Part model, mm, in its own coordinate system. A direction names the side the tool comes from. Give positions to 0.01 mm unless a question says otherwise; leave off trailing zeros. Write each loop counter-clockwise with the first axis right and the second up, starting at its lowest first coordinate (ties: lowest second). Pieces come first, ordered by that corner, then holes.
```python
from build123d import *

# Parameters (mm, degrees)
EXTRUDE_1_DEPTH = 14
EXTRUDE_2_DEPTH = 12
SKETCH_8_W      = 500
SKETCH_8_H      = 12
EXTRUDE_5_DEPTH = 78


with BuildPart() as part:
    # 草图1 → 凸台-拉伸1 (new body)
    with BuildSketch(Plane.XY):
        Polygon((0, 0), (250, 0), (250, 50), (100, 240), (100, 340), (0, 340), (-100, 340), (-100, 240), (-250, 50), (-250, 0), align=None)
    extrude(amount=EXTRUDE_1_DEPTH)

    # 草图6 → 凸台-拉伸2 (add)
    with BuildSketch(Plane.XY.offset(14)):
        Polygon((218.421052632, 90), (-218.421052632, 90), (-250, 50), (-250, 0), (250, 0), (250, 50), align=None)
    extrude(amount=EXTRUDE_2_DEPTH)

    # 草图8 → 凸台-拉伸5 (add)
    with BuildSketch(Plane.XY.offset(26)):
        with Locations((0, 6)):
            Rectangle(SKETCH_8_W, SKETCH_8_H)
    extrude(amount=EXTRUDE_5_DEPTH)


solid = part.part
```
1) Wall check: L1, parallel to Z at x = -83, y = 71.5; L2, parallel to Z at x = -13, y = 316; L3, parallel to Y at x = -206, z = 55. Give the ranges that are in metal, low to high.
Answers follow:
L1: z = 0 to 26
L2: z = 0 to 14
L3: y = 0 to 12
2) Pin check, flat tips, straight feed: pin 1 Ø1 at (x, z) = (176, 24.5) entering from +Y; pin 2 Ø5 at (x, z) = (-182, 45.5) entering from +Y; pin 3 Ø11 at (y, z) = (311, 8.5) entering from -X. Stop position of each tip, or through.
Answers follow:
pin 1: stops at y = 90
pin 2: stops at y = 12
pin 3: stops at x = -100
3) Saw through at C-C, the plane z = 57. Write the cut outline in (x, y).
Answers follow:
outline: (-250, 0) - (250, 0) - (250, 12) - (-250, 12) - close
4) Saw through at D-D, the plane x = -113. Write the cut outline in (y, z), then the cut area to 3 significant figures.
Answers follow:
outline: (0, 0) - (223.53, 0) - (223.53, 14) - (90, 14) - (90, 26) - (12, 26) - (12, 104) - (0, 104) - close
area: 5,150 mm2
5) 3-axis set-ups, long thin cutter, end or side, ignore diameter. For faces 1 (the face through (100, 289, 7)), 2 (the face through (-3, 12, 64)), 3 (the face through (-100, 291, 7)), 4 (the face through (-3, 6, 104)): which of +Z, -Z, +X, -X, +Y, -Y reach the whole face in a straight line?
Answers follow:
face 1: +Z, -Z, +X, +Y
face 2: +Z, +X, -X, +Y
face 3: +Z, -Z, -X, +Y
face 4: +Z, +X, -X, +Y, -Y
6) Saw through at A-A, the plane x = 52. Write the cut outline in (y, z), then the cut area to 3 significant figures.
Answers follow:
outline: (0, 0) - (340, 0) - (340, 14) - (90, 14) - (90, 26) - (12, 26) - (12, 104) - (0, 104) - close
area: 6,780 mm2
7) Saw through at B-B, the plane y = 221. Write the cut outline in (x, z), then the cut area to 3 significant figures.
Answers follow:
outline: (-115, 0) - (115, 0) - (115, 14) - (-115, 14) - close
area: 3,220 mm2
